Check sheet for the modelled part. Datum: model origin and axes. Units: mm. A direction names the side the tool comes from. Give positions to 0.01 mm unless a question says otherwise; leave off trailing zeros. Order: outer loops, then holes, each group sorted by start corner. A loop starts at its lowest first (then second) coordinate and runs counter-clockwise, first axis right, second up.
from build123d import *

# Parameters (mm, degrees)
BOSS_EXTRU_1_DEPTH      = 10
ESQUISSE3_R             = 2
ENL_V_MAT_EXTRU_1_DEPTH = 10
CONG_1_R                = 10
ESQUISSE4_R             = 32.5
ENL_V_MAT_EXTRU_2_DEPTH = 10
ESQUISSE5_R             = 2
ENL_V_MAT_EXTRU_3_DEPTH = 10
ESQUISSE6_W             = 270
ESQUISSE6_H             = 22
ENL_V_MAT_EXTRU_4_DEPTH = 10
ESQUISSE7_R             = 2
ENL_V_MAT_EXTRU_5_DEPTH = 10
ESQUISSE10_R            = 6
ENL_V_MAT_EXTRU_6_DEPTH = 5


with BuildPart() as part:
    # Esquisse2 → Boss.-Extru.1 (new body)
    with BuildSketch(Plane(origin=(0, 0, 0), x_dir=(1, 0, 0), z_dir=(0, 1, 0))):
        Polygon((0, 0), (290, 0), (290, 180), (275, 180), (225, 130), (65, 130), (15, 180), (0, 180), align=None)
    extrude(amount=BOSS_EXTRU_1_DEPTH)

    # Esquisse3 → Enlèv. mat.-Extru.1 (cut)
    with BuildSketch(Plane(origin=(0, 10, 0), x_dir=(1, 0, 0), z_dir=(0, 1, 0))):
        with Locations((10, 10)):
            Circle(ESQUISSE3_R)
        with Locations((280, 10)):
            Circle(ESQUISSE3_R)
    extrude(amount=-ENL_V_MAT_EXTRU_1_DEPTH, mode=Mode.SUBTRACT)

    # Congé1
    cong_1_edges = [part.edges().sort_by_distance(p)[0] for p in [
        (290, 5, 0),
        (0, 5, 0),
    ]]
    fillet(cong_1_edges, radius=CONG_1_R)

    # Esquisse4 → Enlèv. mat.-Extru.2 (cut)
    with BuildSketch(Plane.XZ):
        with Locations((239.106279441, -116.309672248)):
            Circle(ESQUISSE4_R)
        with Locations((179.153264776, -81.942630954)):
            Circle(ESQUISSE4_R)
        with Locations((110.048910395, -82.156407472)):
            Circle(ESQUISSE4_R)
        with Locations((50.309672248, -116.893720559)):
            Circle(ESQUISSE4_R)
    extrude(amount=-ENL_V_MAT_EXTRU_2_DEPTH, mode=Mode.SUBTRACT)

    # Esquisse5 → Enlèv. mat.-Extru.3 (cut)
    with BuildSketch(Plane(origin=(0, 0, 0), x_dir=(-1, 0, 0), z_dir=(0, -1, 0))):
        with Locations((-144.50570114, 101.001110603)):
            Circle(ESQUISSE5_R)
        with Locations((-199.571369329, 115.491017964)):
            Circle(ESQUISSE5_R)
        with Locations((-221.896020418, 76.419161677)):
            Circle(ESQUISSE5_R)
        with Locations((-66.897585359, 77.115673706)):
            Circle(ESQUISSE5_R)
        with Locations((-89.572479932, 115.985316824)):
            Circle(ESQUISSE5_R)
    extrude(amount=-ENL_V_MAT_EXTRU_3_DEPTH, mode=Mode.SUBTRACT)

    # Esquisse6 → Enlèv. mat.-Extru.4 (cut)
    with BuildSketch(Plane(origin=(0, 10, 0), x_dir=(1, 0, 0), z_dir=(0, 1, 0))):
        with Locations((145, 26)):
            Rectangle(ESQUISSE6_W, ESQUISSE6_H)
    extrude(amount=-ENL_V_MAT_EXTRU_4_DEPTH, mode=Mode.SUBTRACT)

    # Esquisse7 → Enlèv. mat.-Extru.5 (cut)
    with BuildSketch(Plane(origin=(0, 10, 0), x_dir=(1, 0, 0), z_dir=(0, 1, 0))):
        with Locations((10, 165)):
            Circle(ESQUISSE7_R)
        with Locations((280, 165)):
            Circle(ESQUISSE7_R)
    extrude(amount=-ENL_V_MAT_EXTRU_5_DEPTH, mode=Mode.SUBTRACT)

    # Esquisse10 → Enlèv. mat.-Extru.6 (cut)
    with BuildSketch(Plane(origin=(0, 10, 0), x_dir=(1, 0, 0), z_dir=(0, 1, 0))):
        with Locations((10, 165)):
            Circle(ESQUISSE10_R)
        with Locations((280, 165)):
            Circle(ESQUISSE10_R)
        with Locations((280, 10)):
            Circle(ESQUISSE10_R)
        with Locations((10, 10)):
            Circle(ESQUISSE10_R)
    extrude(amount=-ENL_V_MAT_EXTRU_6_DEPTH, mode=Mode.SUBTRACT)


solid = part.part
1) Section check C-C, the plane y = 7.5. State how many separate pieces and enclosed holes the cut face has, then the cut area to 3 significant figures.
Recorded:
separate pieces: 1
enclosed holes: 10
area: 22,600 mm2
2) Section check B-B, the plane x = 189.5. Record the cut outline in (y, z).
Recorded:
outline: (0, -130) - (10, -130) - (10, -112.75) - (0, -112.75) - close; (0, -51.13) - (10, -51.13) - (10, -37) - (0, -37) - close; (0, -15) - (10, -15) - (10, 0) - (0, 0) - close
3) Depth check by flat-ended pin: pin 1 Ø19 at (x, z) = (280, -10) entering from +Y; pin 2 Ø2.5 at (x, z) = (199.57, -115.49) entering from +Y (3 decimals); pin 3 Ø6 at (x, y) = (108, 3) entering from -Z; pin 4 Ø9.5 at (x, z) = (10, -165) entering from +Y. Enter the tip coordinate at first touch or a pass-through.
Recorded:
pin 1: stops at y = 10
pin 2: passes through
pin 3: stops at z = -130
pin 4: stops at y = 5
4) Material ranges on L1, parallel to X at y = 8.25, z = -35.5; L2, parallel to X at y = 2.2, z = -165; L3, parallel to Z at x = 65.5, y = 9, recorded low to high.
Recorded:
L1: x = 0 to 10, 280 to 290
L2: x = 0 to 8, 12 to 30, 260 to 278, 282 to 290
L3: z = -88.16 to -78.55, -75.69 to -37, -15 to 0
5) Draft check along Z on faces 1 (the face through (259, 5, -164)), 2 (the face through (10, 5, -26)), 3 (the face through (143, 0, -71)), 4 (the face through (35.45, 4.93, -87.99)). Enter one of: +Z half, -Z half, draft (parallel to the pull), parting line (faces both ways), or undercut.
Recorded:
face 1: -Z half
face 2: undercut
face 3: draft
face 4: undercut
6) Section check A-A, the plane z = -95.5. Record the cut outline in (x, y).
Recorded:
outline: (0, 0) - (25.84, 0) - (25.84, 10) - (0, 10) - close; (74.78, 0) - (80.41, 0) - (80.41, 10) - (74.78, 10) - close; (139.68, 0) - (149.62, 0) - (149.62, 10) - (139.68, 10) - close; (208.69, 0) - (214.14, 0) - (214.14, 10) - (208.69, 10) - close; (264.07, 0) - (290, 0) - (290, 10) - (264.07, 10) - close
7) Set-up check for faces 5 (the face through (31, 5, -164)), 6 (the face through (8.699, 7.535, -159.143)), 7 (the face through (8, 5, -180)), 8 (the face through (280, 5, -26)): record each of +Z, -Z, +X, -X, +Y, -Y from which the full face is reachable in a straight line by a thin tool's end or side.
Recorded:
face 5: -Z, +Y, -Y
face 6: +Y
face 7: -Z, +X, -X, +Y, -Y
face 8: +Y, -Y
8) Section check D-D, the plane z = -142. Record the cut outline in (x, y).
Recorded:
outline: (0, 0) - (29.67, 0) - (29.67, 10) - (0, 10) - close; (259.01, 0) - (290, 0) - (290, 10) - (259.01, 10) - close
